Read the model definition and answer for the solid it produces. Units are mm, in the model's axes. A direction names the side the tool comes from. Give positions to 0.01 mm unless a question says otherwise; leave off trailing zeros. Write each loop counter-clockwise with the first axis right and the second up, starting at its lowest first coordinate (ties: lowest second). Pieces come first, ordered by that corner, then holes. Notation, with made-up numbers: (-29.5, 28.25) -> (0.5, 28.25) arc R28 cw to (0.5, 50.25) -> close; hole circle Ø1 at (-20.75, 21.25). An arc over 180 degrees is marked (long way). Use a Markdown table: item, result.
from build123d import *

# Parameters (mm, degrees)
F0_W        = 12.7
F0_H        = 6.35
F0_W_2      = 19.05
F0_H_2      = 187.325
F0_H_3      = 19.05
F0_R        = 1.5875
F0_W_3      = 209.55
F1_DEPTH    = 6.35
F2_R        = 9.525
F3_T1_DEPTH = 31.75


# Not quite as in the source:
# - a fillet or chamfer that OpenCascade refuses, or shapes differently, is made with other operations: its cross-section is extruded or revolved along the edge and cut away or added
# - a length typed as a fraction of an inch, garbled in the dataset ("3 / 203.2 mm" for 3/8 in), is restored


with BuildPart() as f1:
    # F0 (on Top) → F1 (new body)
    with BuildSketch(Plane.XY):
        with Locations((-254, -190.5)):
            Rectangle(F0_W, F0_H)
        with Locations((-238.125, -190.5)):
            Rectangle(F0_W_2, F0_H)
        with Locations((-238.125, -93.6625)):
            Rectangle(F0_W_2, F0_H_2)
        with Locations((-238.125, 9.525)):
            Rectangle(F0_W_2, F0_H_3)
        with Locations((-238.125, 9.525)):
            Circle(F0_R, mode=Mode.SUBTRACT)
        with Locations((-123.825, 9.525)):
            Rectangle(F0_W_3, F0_H_3)
        with Locations((-9.525, 9.525)):
            Rectangle(F0_W_2, F0_H_3)
        with Locations((-9.525, 9.525)):
            Circle(F0_R, mode=Mode.SUBTRACT)
        with Locations((-9.525, -93.6625)):
            Rectangle(F0_W_2, F0_H_2)
        with Locations((-9.525, -190.5)):
            Rectangle(F0_W_2, F0_H)
        with Locations((-25.4, -190.5)):
            Rectangle(F0_W, F0_H)
    extrude(amount=F1_DEPTH)

    # F2
    f2_edges = [f1.edges().sort_by_distance(p)[0] for p in [
        (0, 19.05, 3.175),
        (-247.65, 19.05, 3.175),
    ]]
    fillet(f2_edges, radius=F2_R)

    # F3: fillet of radius 5.08 on 4 edges, made by hand

    # F3_s2 → F3_t1 (cut)
    with BuildSketch(Plane.XY.offset(-12.7)):
        with BuildLine():
            ThreePointArc((-255.27, -187.325), (-258.8621024484, -188.8128975516), (-260.35, -192.405))
            Line((-260.35, -192.405), (-260.35, -187.325))
            Line((-260.35, -187.325), (-255.27, -187.325))
        make_face()
        with BuildLine():
            ThreePointArc((-31.75, -192.405), (-30.2621024484, -188.8128975516), (-26.67, -187.325))
            Line((-26.67, -187.325), (-31.75, -187.325))
            Line((-31.75, -187.325), (-31.75, -192.405))
        make_face()
        with BuildLine():
            ThreePointArc((-260.35, -188.595), (-258.8621024484, -192.1871024484), (-255.27, -193.675))
            Line((-255.27, -193.675), (-260.35, -193.675))
            Line((-260.35, -193.675), (-260.35, -188.595))
        make_face()
        with BuildLine():
            ThreePointArc((-26.67, -193.675), (-30.2621024484, -192.1871024484), (-31.75, -188.595))
            Line((-31.75, -188.595), (-31.75, -193.675))
            Line((-31.75, -193.675), (-26.67, -193.675))
        make_face()
    extrude(amount=F3_T1_DEPTH, mode=Mode.SUBTRACT)


solid = f1.part
Item 1: A cutting plane is placed at C-C (x = -22.5). Give the vertices of the cut face in (y, z) (3 decimals).
Return value:
| item | result |
|---|---|
| outline | (-193.675, 0) -> (-187.325, 0) -> (-187.325, 6.35) -> (-193.675, 6.35) -> close; (0, 0) -> (19.05, 0) -> (19.05, 6.35) -> (0, 6.35) -> close |
Item 2: A tool of negligible diameter and unlimited length cuts with its end or side. For faces 5 (the face through (-247.65, -88, 3)), 6 (the face through (-228.6, -98, 3)), 7 (the face through (-2.72, 16.19, 3.22)), from which of +Z, -Z, +X, -X, +Y, -Y can it reach the whole face along a straight path? Write none if from no direction.
Return value:
| item | result |
|---|---|
| face 5 | +Z, -Z, -X, +Y |
| face 6 | +Z, -Z, -Y |
| face 7 | +Z, -Z, +X, +Y |
Item 3: Each of these flat-tipped pins is pushed along its axis until it touches: P1, Ø1, axis at x = -91, z = 0.5, coming from the -Y side; P2, Ø3, axis at y = -95.5, z = 2.5, coming from the -X side; P3, Ø3, axis at x = -238.125, y = 9.525, coming from the -Z side. Where does it stop, or does it pass through?
Return value:
| item | result |
|---|---|
| P1 | y = 0 |
| P2 | x = -247.65 |
| P3 | through |
Item 4: Straight lines are drawn through the part: line 1 along X through (y, z) = (-135, 5); line 2 along Y through (x, z) = (-46, 1.5); line 3 along X through (y, z) = (2.5, 0.5). For each, find the intervals that lie inside material, in ascending order. Write a range as [from, to].
Return value:
| item | result |
|---|---|
| line 1 | [-247.65, -228.6], [-19.05, 0] |
| line 2 | [0, 19.05] |
| line 3 | [-247.65, 0] |
Item 5: A cutting plane is placed at B-B (y = -62.5). Give the vertices of the cut face in (x, z).
Return value:
| item | result |
|---|---|
| outline | (-247.65, 0) -> (-228.6, 0) -> (-228.6, 6.35) -> (-247.65, 6.35) -> close; (-19.05, 0) -> (0, 0) -> (0, 6.35) -> (-19.05, 6.35) -> close |
Item 6: A cutting plane is placed at D-D (y = 3). Give the vertices of the cut face in (x, z).
Return value:
| item | result |
|---|---|
| outline | (-247.65, 0) -> (0, 0) -> (0, 6.35) -> (-247.65, 6.35) -> close |
Item 7: For a pull along Y with two mould halves and no side action, classify faces 1 (the face through (-244.79, 16.33, 3.22)), 2 (the face through (-19.05, -92, 3)), 3 (the face through (-23, -187.325, 3)), 4 (the face through (-121, 8, 6.35)) as +Y half, -Y half, draft (parallel to the pull), parting line (faces both ways), or undercut.
Return value:
| item | result |
|---|---|
| face 1 | +Y half |
| face 2 | undercut |
| face 3 | undercut |
| face 4 | draft |
Item 8: A cutting plane is placed at A-A (z = 1). Count the separate pieces of the cut face and the enclosed holes in it, then the cut area to 3 significant figures.
Return value:
| item | result |
|---|---|
| separate pieces | 1 |
| enclosed holes | 2 |
| area | 12,200 mm^2 |
